Read the model definition and answer for the solid it produces. Units are mm, in the model's axes. A direction names the side the tool comes from. Give positions to 0.01 mm unless a question says otherwise; leave off trailing zeros. Write each loop counter-clockwise with the first axis right and the second up, starting at its lowest first coordinate (ties: lowest second). Pieces come first, ordered by that corner, then holes.
```python
from build123d import *

# Parameters (mm, degrees)
PAD_DEPTH           = 2.4
SKETCH002_R         = 1.2
PAD001_DEPTH        = 3
SKETCH003_R         = 4.3
SKETCH003_R_2       = 2.6
PAD002_DEPTH        = 3
PAD003_DEPTH        = 2
LINEARPATTERN_COUNT = 2
LINEARPATTERN_PITCH = 5
SKETCH006_R         = 1.8
POCKET_DEPTH        = 0.6


with BuildPart() as part:
    # Sketch → Pad (new body)
    with BuildSketch(Plane.XY):
        Polygon((-26.4, 8.7), (26.4, 8.7), (35.1, 0), (26.4, -8.7), (-26.4, -8.7), (-35.1, 0), align=None)
    extrude(amount=PAD_DEPTH)

    # Sketch002 → Pad001 (join)
    with BuildSketch(Plane.YZ.offset(15)):
        with BuildLine():
            Line((-6, 2.4), (6, 2.4))
            Line((6, 2.4), (4.2734913846, 17.8767298872))
            ThreePointArc((4.2734913846, 17.8767298872), (0, 21.7), (-4.2734913846, 17.8767298872))
            Line((-6, 2.4), (-4.2734913846, 17.8767298872))
        make_face()
        with Locations((0, 17.4)):
            Circle(SKETCH002_R, mode=Mode.SUBTRACT)
    extrude(amount=PAD001_DEPTH)

    # Sketch003 (on Face12 of Pad001) → Pad002 (join)
    with BuildSketch(Plane(origin=(15, 0, 0), x_dir=(0, -1, 0), z_dir=(-1, 0, 0))):
        with Locations((0, 17.4)):
            Circle(SKETCH003_R)
        with Locations((0, 17.4)):
            Circle(SKETCH003_R_2, mode=Mode.SUBTRACT)
    extrude(amount=PAD002_DEPTH)

    # Sketch005 → Pad003 (join)
    with BuildSketch(Plane.XZ.offset(1.5)):
        Polygon((10.2, 2.4), (15, 13.2), (15, 2.4), align=None)
        Polygon((18, 13.2), (18, 2.4), (22.8, 2.4), align=None)
    pad003 = extrude(amount=PAD003_DEPTH)

    # LinearPattern: Pad003 ×2
    with Locations(*[(0, i * LINEARPATTERN_PITCH, 0) for i in range(1, LINEARPATTERN_COUNT)]):
        add(pad003)

    # Sketch006 (on Face10 of LinearPattern) → Pocket (cut)
    with BuildSketch(Plane.YZ.offset(18)):
        with Locations((0, 17.4)):
            Circle(SKETCH006_R)
    extrude(amount=-POCKET_DEPTH, mode=Mode.SUBTRACT)


solid = part.part
```
Item 1: Which of the six approach directions +Z, -Z, +X, -X, +Y, -Y give full straight-line access (tool end or side, diameter ignored) to faces 4 (the cylindrical face through (14, 1, 15)), 5 (the flat face through (14, 3.5, 5)), 6 (the flat face through (18, 0, 12)), 7 (the flat face through (14, -3.5, 5))?
Result set:
face 4: -X
face 5: -X, +Y
face 6: +Z, +X
face 7: -X, -Y
Item 2: Section B-B (z = 12) is taken. Write down the section's boundary in (x, y).
Result set:
outline: (14.47, -3.5) - (15, -3.5) - (15, -4.93) - (18, -4.93) - (18, -3.5) - (18.53, -3.5) - (18.53, -1.5) - (18, -1.5) - (18, 1.5) - (18.53, 1.5) - (18.53, 3.5) - (18, 3.5) - (18, 4.93) - (15, 4.93) - (15, 3.5) - (14.47, 3.5) - (14.47, 1.5) - (15, 1.5) - (15, -1.5) - (14.47, -1.5) - close
Item 3: Find the intervals of material crossed by line 1 along Z through (x, y) = (14.05, 0); line 2 along Y through (x, z) = (12, 5); line 3 along Z through (x, y) = (-11, -7.5), in increasing order.
Result set:
line 1: z = 0 to 2.4, 13.1 to 14.8, 20 to 21.7
line 2: y = -3.5 to -1.5, 1.5 to 3.5
line 3: z = 0 to 2.4
Item 4: Determine the mould class of faces 1 (the flat face through (20.434, -2.486, 7.724)), 2 (the flat face through (17.4, 0, 16)), 3 (the flat face through (19, -3.5, 5)) for opening direction Z: pulls with the +Z half, pulls with the -Z half, needs draft (parallel to the pull), parting line crosses it, or undercut.
Result set:
face 1: pulls with the +Z half
face 2: undercut
face 3: needs draft
Item 5: Section A-A (x = 11) is taken. Write down the section's boundary in (y, z), and give its area (3 significant figures).
Result set:
outline: (-8.7, 0) - (8.7, 0) - (8.7, 2.4) - (3.5, 2.4) - (3.5, 4.2) - (1.5, 4.2) - (1.5, 2.4) - (-1.5, 2.4) - (-1.5, 4.2) - (-3.5, 4.2) - (-3.5, 2.4) - (-8.7, 2.4) - close
area: 49.0 mm2
Item 6: Section C-C (x = -7) is taken. Write down the section's boundary in (y, z).
Result set:
outline: (-8.7, 0) - (8.7, 0) - (8.7, 2.4) - (-8.7, 2.4) - close
Item 7: Each of these flat-tipped pins is pushed along its axis until it touches: pin 1 Ø2 at (x, y) = (-27, 7) entering from +Z; pin 2 Ø5 at (y, z) = (-3.5, 8.5) entering from +X; pin 3 Ø1.5 at (y, z) = (7, 14.5) entering from -X; pin 4 Ø5.5 at (x, z) = (21, 8) entering from -Y. Where does it stop, or does it pass through?
Result set:
pin 1: stops at z = 2.4
pin 2: stops at x = 21.2
pin 3: passes through
pin 4: stops at y = -3.5
